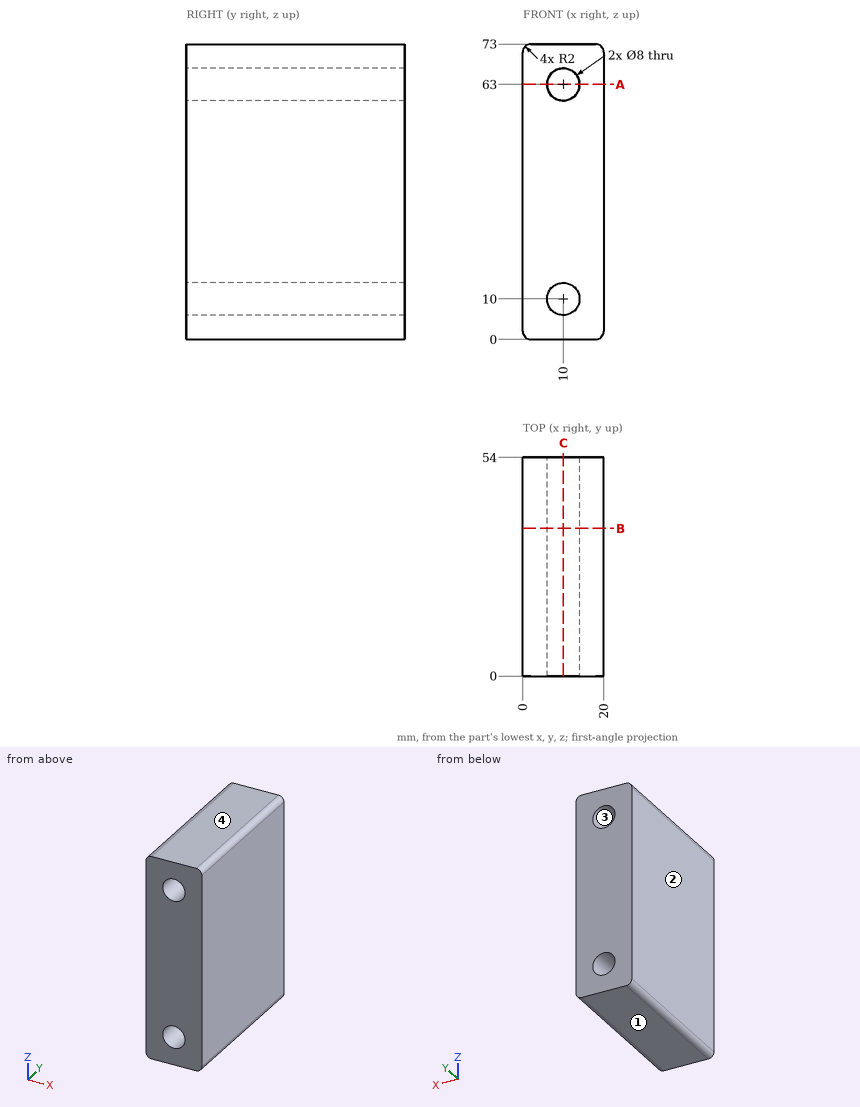
Here's the drawing with two shaded views (mm, measured from the low corner). I have some questions. Give positions to 0.01 mm unless a question says otherwise; leave off trailing zeros. Loops run counter-clockwise (first coordinate to the right, second up) from the corner with the lowest first, then second, coordinate; pieces in that order, holes last. Notation, with made-up numbers: (-28, 43.5) - (-21, 43.5) arc R26 cw to (-21, 59.5) - close; hole circle Ø6 at (39, 40.25). An arc over 180 degrees is marked (long way). Answer in a Markdown table with one row per item. Add a question column.
Q1. If we section it at B-B (y = 36.5): List the corners of the cut face in (x, z) for me, plus the area to 3 significant figures.
Q2. If we section it at C-C (x = 10): List the corners of the cut face in (y, z) for me.
Q3. We'd pull the mould along Z, two halves only. Please class the marked faces 1, 2, 3 and 4: +Z half, -Z half, draft (parallel to the pull), parting line (faces both ways), or undercut.
Q4. If we section it at A-A (z = 63): List the corners of the cut face in (x, y) for me.
Q5. For pin 1 (3 mm diameter, centred on x = 10, y = 16.5, fed in from -Z); pin 2 (5 mm diameter, centred on x = 10, z = 10, fed in from +Y), each with a flat end and sliding along its axis, tell me the tip position at first contact or that it passes through.
Q6. Please list where these lines run through material, in increasing order: L1, parallel to Z at x = 10, y = 19; L2, parallel to X at y = 20, z = 63; L3, parallel to Z at x = 7.75, y = 32.5. Write a range as from..to.
The answers:
| question | item | result |
|---|---|---|
| 1 | outline | (0, 2) arc R2 ccw to (2, 0) - (18, 0) arc R2 ccw to (20, 2) - (20, 71) arc R2 ccw to (18, 73) - (2, 73) arc R2 ccw to (0, 71) - close; hole circle Ø8 at (10, 10); hole circle Ø8 at (10, 63) |
| 1 | area | 1,360 mm^2 |
| 2 | outline | (0, 0) - (54, 0) - (54, 6) - (0, 6) - close; (0, 14) - (54, 14) - (54, 59) - (0, 59) - close; (0, 67) - (54, 67) - (54, 73) - (0, 73) - close |
| 3 | face 1 | -Z half |
| 3 | face 2 | draft |
| 3 | face 3 | undercut |
| 3 | face 4 | +Z half |
| 4 | outline | (0, 0) - (6, 0) - (6, 54) - (0, 54) - close; (14, 0) - (20, 0) - (20, 54) - (14, 54) - close |
| 5 | pin 1 | stops at z = 0 |
| 5 | pin 2 | passes through |
| 6 | L1 | z = 0..6, 14..59, 67..73 |
| 6 | L2 | x = 0..6, 14..20 |
| 6 | L3 | z = 0..6.69, 13.31..59.69, 66.31..73 |
